Could you check a few things on this model? Use its own coordinates, in mm. Face numbers are marked on the shaded views. A direction names the side the tool comes from. Give positions to 0.01 mm unless a question says otherwise; leave off trailing zeros. Loops run counter-clockwise (first coordinate to the right, second up) from the corner with the lowest first, then second, coordinate; pieces in that order, holes last. Notation, with made-up numbers: M 34,-14 L 45,-14 A6 cw 45,-7 Z; hole C -11,70.25 d10. An arc over 180 degrees is marked long. Answer in a Markdown table with one row per item. Add a question column.
```python
from build123d import *

# Parameters (mm, degrees)
F0_R      = 12.5
F1_DEPTH  = 30
F2_DEPTH  = 21.2
F3_R      = 2
F4_R      = 2
F5_R      = 2
F6_R      = 2
F7_R      = 13.25
F7_R_2    = 12.5
F8_DEPTH  = 3.5
F7_R_3    = 18
F7_R_4    = 17.5
F10_DEPTH = 0.1


# Not quite as in the source:
# - the program builds the solid bodies; features that only make, move or delete a surface that nothing else refers to are left out


with BuildPart() as f1:
    # F0 (on Front) → F1 (new body)
    with BuildSketch(Plane.XZ):
        with Locations((14, 0)):
            Circle(F0_R)
    extrude(amount=F1_DEPTH)

    # F0 (on Front) → F2 (join)
    with BuildSketch(Plane.XZ):
        Polygon((30.2, -21), (30.2, 0), (30.2, 21), (-30.2, 21), (-30.2, -21), align=None)
        with Locations((14, 0)):
            Circle(F0_R, mode=Mode.SUBTRACT)
    extrude(amount=F2_DEPTH)

    # F3
    f3_edges = [f1.edges().sort_by_distance(p)[0] for p in [
        (-30.2, -10.6, 21),
    ]]
    fillet(f3_edges, radius=F3_R)

    # F4
    f4_edges = [f1.edges().sort_by_distance(p)[0] for p in [
        (30.2, -10.6, 21),
    ]]
    fillet(f4_edges, radius=F4_R)

    # F5
    f5_edges = [f1.edges().sort_by_distance(p)[0] for p in [
        (-30.2, -10.6, -21),
    ]]
    fillet(f5_edges, radius=F5_R)

    # F6
    f6_edges = [f1.edges().sort_by_distance(p)[0] for p in [
        (30.2, -10.6, -21),
    ]]
    fillet(f6_edges, radius=F6_R)

    # F7 (on face) → F8 (join)
    with BuildSketch(Plane.XZ.offset(30)):
        with Locations((14, 0)):
            Circle(F7_R)
        with Locations((14, 0)):
            Circle(F7_R_2, mode=Mode.SUBTRACT)
    extrude(amount=-F8_DEPTH)

    # F7 (on face) → F10 (join)
    with BuildSketch(Plane.XZ.offset(30)):
        with Locations((14, 0)):
            Circle(F7_R_3)
        with Locations((14, 0)):
            Circle(F7_R_4, mode=Mode.SUBTRACT)
        with Locations((14, 0)):
            Circle(F7_R_4)
        with Locations((14, 0)):
            Circle(F7_R, mode=Mode.SUBTRACT)
    extrude(amount=-F10_DEPTH)


solid = f1.part
```
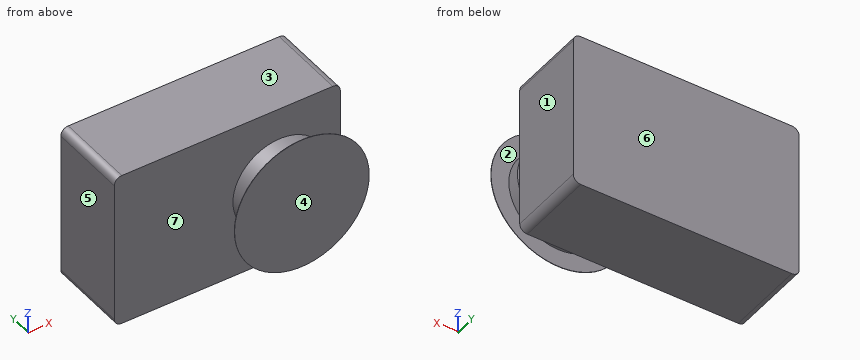
Item 1: Suppose I cut it at B-B (y = -9). List the corners of the cut face in (x, z) for me, then the cut area to 3 significant figures.
Item 2: For P1, Ø3, axis at y = -23.5, z = -4.5, coming from the +X side; P2, Ø10.5, axis at y = -6.5, z = -2.5, coming from the +X side; P3, Ø5, axis at x = -5.5, y = -25.5, coming from the +Z side; P4, Ø6, axis at y = -25.5, z = 8.5, coming from the -X side, each with a flat end and sliding along its axis, tell me the tip position at first contact or that it passes through.
Item 3: If we mould it in two halves opening along Y, with no side actions, what happens to the marked faces 4, 5, 6 and 7? For each: +Y half, -Y half, draft (parallel to the pull), parting line (faces both ways), or undercut.
Item 4: I need wall thicknesses on L1, parallel to Y at x = 5, z = -9; L2, parallel to Y at x = -20.5, z = 2; L3, parallel to X at y = -13, z = -16. Which ranges of each line are inside material? Lowest first, please.
Item 5: Suppose I cut it at C-C (x = 14). List the corners of the cut face in (y, z) for me, then the cut area to 3 significant figures.
Item 6: For the marked faces 1, 2 and 3, which set-ups out of +Z, -Z, +X, -X, +Y, -Y let a thin tool reach every point of the face, with its end or its side?
Item 7: Suppose I cut it at D-D (z = 0). List the corners of the cut face in (x, y) for me, then the cut area to 3 significant figures.
Item 8: Suppose I cut it at A-A (z = -16.5). List the corners of the cut face in (x, y) for me.
Values found:
| question | item | result |
|---|---|---|
| 1 | outline | M -30.2,-19 A2 ccw -28.2,-21 L 28.2,-21 A2 ccw 30.2,-19 L 30.2,19 A2 ccw 28.2,21 L -28.2,21 A2 ccw -30.2,19 Z |
| 1 | area | 2,530 mm² |
| 2 | P1 | x = 26.13 |
| 2 | P2 | x = 30.2 |
| 2 | P3 | through |
| 2 | P4 | x = 2.03 |
| 3 | face 4 | -Y half |
| 3 | face 5 | draft |
| 3 | face 6 | +Y half |
| 3 | face 7 | undercut |
| 4 | L1 | -30 to -26.5, -21.2 to 0 |
| 4 | L2 | -21.2 to 0 |
| 4 | L3 | -30.2 to 30.2 |
| 5 | outline | M -30,-18 L -29.9,-18 L -29.9,-13.25 L -26.5,-13.25 L -26.5,-12.5 L -21.2,-12.5 L -21.2,-21 L 0,-21 L 0,21 L -21.2,21 L -21.2,12.5 L -26.5,12.5 L -26.5,13.25 L -29.9,13.25 L -29.9,18 L -30,18 Z |
| 5 | area | 1,120 mm² |
| 6 | face 1 | +Z, -Z, +X, +Y |
| 6 | face 2 | none |
| 6 | face 3 | +Z, +X, -X, +Y, -Y |
| 7 | outline | M -30.2,-21.2 L 1.5,-21.2 L 1.5,-26.5 L 0.75,-26.5 L 0.75,-29.9 L -4,-29.9 L -4,-30 L 32,-30 L 32,-29.9 L 27.25,-29.9 L 27.25,-26.5 L 26.5,-26.5 L 26.5,-21.2 L 30.2,-21.2 L 30.2,0 L -30.2,0 Z |
| 7 | area | 1,510 mm² |
| 8 | outline | M -30.2,-21.2 L 30.2,-21.2 L 30.2,0 L -30.2,0 Z; M 6.81,-30 L 21.19,-30 L 21.19,-29.9 L 6.81,-29.9 Z |
